from build123d import *

# Parameters (mm, degrees)
F0_W     = 94.794575125
F0_H     = 66.0311877728
F1_DEPTH = 229.37163
F2_W     = 367.8625924513
F2_H     = 239.847317338
F2_W_2   = 389.3495500088
F2_H_2   = 207.6520100236
F2_W_3   = 314.4028186798
F2_H_3   = 402.6826024055
F2_W_4   = 43.3726906776
F2_H_4   = 9.1089755297
F2_W_5   = 145.0487077236
F2_H_5   = 58.66086483
F2_H_6   = 143.2274132967
F2_W_6   = 144.3722844124
F3_DEPTH = 89.50501


with BuildPart() as f1:
    # F0 (on Front) → F1 (new body)
    with BuildSketch(Plane.XZ):
        with Locations((14.3123473972, 155.8356285095)):
            Rectangle(F0_W, F0_H)
    extrude(amount=F1_DEPTH)

    # F2 (on Front) → F3 (join)
    with BuildSketch(Plane.XZ):
        with Locations((-170.1408275403, -119.923658669)):
            Rectangle(F2_W, F2_H)
        Polygon((-354.0721237659, 0), (13.7904686853, 0), (287.5355780125, 0), (287.5355780125, 207.2783261538), (287.5355780125, 236.5134656429), (287.5355780125, 397.2084522247), (-39.6693050861, 397.2084522247), (-354.0721237659, 397.2084522247), (-354.0721237659, 293.8325405121), (-354.0721237659, 86.1805304885), align=None)
        with Locations((-548.7468987703, 190.0065355003)):
            Rectangle(F2_W_2, F2_H_2)
        Polygon((287.5355780125, 236.5134656429), (287.5355780125, 207.2783261538), (326.2129127979, 207.2783261538), (326.2129127979, 225.2303659916), (326.2129127979, 234.3393415213), (326.2129127979, 236.5134656429), align=None)
        with Locations((-196.870714426, 598.5497534275)):
            Rectangle(F2_W_3, F2_H_3)
        with Locations((347.8992581367, 229.7848537564)):
            Rectangle(F2_W_4, F2_H_4)
        with Locations((442.1099573374, 229.7848537564)):
            Rectangle(F2_W_5, F2_H_4)
        with Locations((442.1099573374, 195.8999335766)):
            Rectangle(F2_W_5, F2_H_5)
        with Locations((442.1099573374, 305.9530481696)):
            Rectangle(F2_W_5, F2_H_6)
        with Locations((586.8204534054, 229.7848537564)):
            Rectangle(F2_W_6, F2_H_4)
    extrude(amount=F3_DEPTH)


solid = f1.part
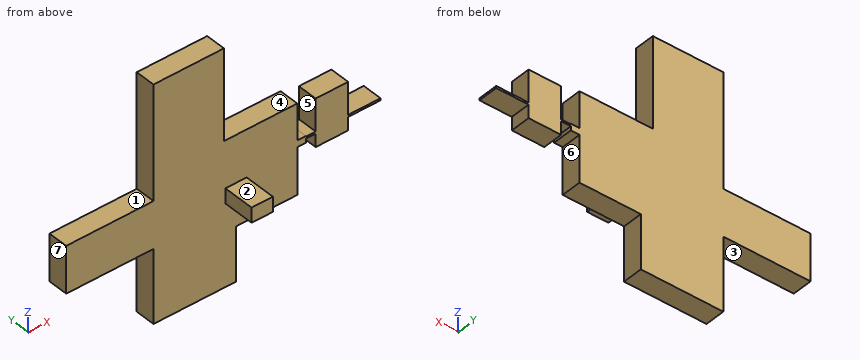
Geometry: final body of the model. Coordinates: model frame, mm. Face numbers are marked on the shaded views. A direction names the side the tool comes from. Round coordinates to 2 decimals unless told otherwise and drop trailing zeros. Loops run counter-clockwise (first coordinate to the right, second up) from the corner with the lowest first, then second, coordinate; pieces in that order, holes last. Notation, with made-up numbers: M 73,76 L 120,76 A16 ccw 120,106 Z; hole C -18,-26.5 d8. An arc over 180 degrees is marked long. Put each result on its own line as item: value. Start each with the question number.
(1) Section query A-A (z = 333). Return loops of the section in (x, y), then the cut area to 3 significant figures.
(2) Section query B-B (x = 46). Return loops of the section in (y, z).
(3) Set-up query: the marked faces 1, 2 and 3. Return all of +Z, -Z, +X, -X, +Y, -Y with unobstructed straight access to the full face (end or side cutting, diameter ignored); none if empty.
(4) Material intervals for line 1 along Y through (x, z) = (-90, -46.5); line 2 along X through (y, z) = (-38.5, 122); line 3 along X through (y, z) = (-68.5, 622), sorted ascending. Write a range as [from, to].
(5) Section query D-D (z = -87.5). Return loops of the section in (x, y).
(6) Draft query along X for the marked faces 4, 5, 6 and 7. Return one class per face: +X half, -X half, draft (parallel to the pull), parting line (faces both ways), or undercut.
(7) Section query C-C (y = -17). Return loops of the section in (x, z).
(8) Contact query for flat-ended pins moving along their axis: pin 1 Ø1.7 at (y, z) = (-40, 236) entering from +X; pin 2 Ø3 at (x, y) = (-5, -137) entering from -Z; pin 3 Ø3 at (y, z) = (-27, 607) entering from -X. Output: stop coordinate, or through.
Findings below:
1. outline: M -354.07,-89.51 L 287.54,-89.51 L 287.54,0 L -354.07,0 Z; M 369.59,-89.51 L 514.63,-89.51 L 514.63,0 L 369.59,0 Z
1. area: 70,400 mm2
2. outline: M -229.37,122.82 L -89.51,122.82 L -89.51,0 L 0,0 L 0,397.21 L -89.51,397.21 L -89.51,188.85 L -229.37,188.85 Z
3. face 1: +Z, -X, +Y, -Y
3. face 2: +Z, +X, -X, -Y
3. face 3: -Z, -X, +Y, -Y
4. line 1: y = [-89.51, 0]
4. line 2: x = [-743.42, 287.54]
4. line 3: x = [-354.07, -39.67]
5. outline: M -354.07,-89.51 L 13.79,-89.51 L 13.79,0 L -354.07,0 Z
6. face 4: draft
6. face 5: undercut
6. face 6: undercut
6. face 7: -X half
7. outline: M -743.42,86.18 L -354.07,86.18 L -354.07,-239.85 L 13.79,-239.85 L 13.79,0 L 287.54,0 L 287.54,207.28 L 326.21,207.28 L 326.21,225.23 L 369.59,225.23 L 369.59,166.57 L 514.63,166.57 L 514.63,225.23 L 659.01,225.23 L 659.01,234.34 L 514.63,234.34 L 514.63,377.57 L 369.59,377.57 L 369.59,234.34 L 326.21,234.34 L 326.21,236.51 L 287.54,236.51 L 287.54,397.21 L -39.67,397.21 L -39.67,799.89 L -354.07,799.89 L -354.07,293.83 L -743.42,293.83 Z
8. pin 1: stops at x = 514.63
8. pin 2: stops at z = 122.82
8. pin 3: stops at x = -354.07
